Check sheet for the modelled part. Datum: model origin and axes. Units: mm. A direction names the side the tool comes from. Coordinates: 2 decimals unless noted, no trailing zeros. Write each loop counter-clockwise with the first axis right and the second up, starting at its lowest first coordinate (ties: lowest second). Pieces come first, ordered by that corner, then holes. Notation, with made-up numbers: (-28, 69) - (23, 69) arc R23 cw to (23, 103) - close; hole circle Ø10 at (15.5, 3.25). An arc over 180 degrees is marked (long way). Write each question's results on one line, items separated by ' | '.
from build123d import *

# Parameters (mm, degrees)
SKETCH_R           = 25
SKETCH_R_2         = 2.7
PAD_DEPTH          = 10
POCKET_DEPTH       = 3.5
POCKET001_DEPTH    = 152.829569
POLARPATTERN_COUNT = 16
SKETCH003_R        = 20
SKETCH003_R_2      = 2.7
PAD001_DEPTH       = 10


with BuildPart() as part:
    # Sketch → Pad (new body)
    with BuildSketch(Plane.XY):
        Circle(SKETCH_R)
        Circle(SKETCH_R_2, mode=Mode.SUBTRACT)
    extrude(amount=PAD_DEPTH)

    # Sketch001 (on DatumPlane) → Pocket (cut)
    with BuildSketch(Plane.XY.offset(10)):
        Polygon((5.5, -3.175426), (5.5, 3.175426), (0, 6.350853), (-5.5, 3.175426), (-5.5, -3.175426), (0, -6.350853), align=None)
    extrude(amount=-POCKET_DEPTH, mode=Mode.SUBTRACT)

    # Sketch002 (on DatumPlane) → Pocket001 (cut, through all)
    with BuildSketch(Plane.XY.offset(10)):
        with BuildLine():
            Line((24.148146, 6.470476), (23.298954, 3.067366))
            Line((23.298954, 3.067366), (25, 0))
            ThreePointArc((25, 0), (26.776409, 3.525181), (24.148146, 6.470476))
        make_face()
    pocket001 = extrude(amount=-POCKET001_DEPTH, mode=Mode.SUBTRACT)

    # PolarPattern: Pocket001 ×16 about axis
    polarpattern_axis = Axis((0, 0, 10), (0, 0, 1))
    for i in range(1, POLARPATTERN_COUNT):
        add(pocket001.rotate(polarpattern_axis, i * 360 / POLARPATTERN_COUNT), mode=Mode.SUBTRACT)

    # Sketch003 (on Face5 of PolarPattern) → Pad001 (join)
    with BuildSketch(Plane(origin=(0, 0, 0), x_dir=(1, 0, 0), z_dir=(0, 0, -1))):
        Circle(SKETCH003_R)
        Circle(SKETCH003_R_2, mode=Mode.SUBTRACT)
    extrude(amount=PAD001_DEPTH)


solid = part.part
1. Go/stop test with flat-tipped pins: pin 1 (6 mm diameter, centred on x = 7, z = 3.5, fed in from -Y); pin 2 (3 mm diameter, centred on x = -0.5, z = -6, fed in from -Y); pin 3 (3.5 mm diameter, centred on x = 0, y = 3, fed in from +Z); pin 4 (3 mm diameter, centred on x = 0, y = 0, fed in from +Z). Record where each tip stops, or that it passes through.
Values follow:
pin 1: stops at y = -24.15 | pin 2: stops at y = -20 | pin 3: stops at z = 6.5 | pin 4: passes through
2. Access from +Z, -Z, +X, -X, +Y, -Y to the whole of each face (thin tool, end or side, straight path). Record for faces 1 (the flat face through (-4.65, -23.76, 5.07)), 2 (the flat face through (23.73, 4.79, 5.07)), 3 (the flat face through (-5.5, 0, 8)), 4 (the flat face through (4.65, 23.76, 5.07)), 5 (the flat face through (-23.76, 4.65, 5.07)).
Values follow:
face 1: +Z, -Z, -Y | face 2: +Z, -Z, +X | face 3: +Z | face 4: +Z, -Z, +Y | face 5: +Z, -Z, -X
3. Sectioned sample at B-B (y = 11). Record the cut outline in (x, z).
Values follow:
outline: (-22.45, 0) - (-16.7, 0) - (-16.7, -10) - (16.7, -10) - (16.7, 0) - (21.29, 0) - (21.29, 10) - (-22.45, 10) - close
4. Material ranges on L1, parallel to X at y = 0, z = -5.75; L2, parallel to Y at x = 0, z = 0.75, recorded low to high. Write a range as [from, to].
Values follow:
L1: x = [-20, -2.7], [2.7, 20] | L2: y = [-25, -2.7], [2.7, 25]
5. Draft check along X on faces 6 (the flat face through (23.76, -4.65, 5.07)), 7 (the flat face through (-22.895, 7.8, 5.07)), 8 (the flat face through (4.79, -23.73, 5.07)). Enter one of: pulls with the +X half, pulls with the -X half, needs draft (parallel to the pull), parting line crosses it, or undercut.
Values follow:
face 6: pulls with the +X half | face 7: pulls with the -X half | face 8: undercut
6. Sectioned sample at A-A (z = -4). Record the cut outline in (x, y).
Values follow:
outline: circle Ø40 at (0, 0); hole circle Ø5.4 at (0, 0)
